from build123d import *

# Parameters (mm, degrees)
SKETCH_1_R             = 5.25
SM_BASE_FLANGE_1_DEPTH = 6


# Sheet-metal steps are written as plain solids
with BuildPart() as part:
    # Sketch 1 → Базовая кромка1 (new body)
    with BuildSketch(Plane.XY):
        Polygon((-41, -132.5), (-56, -117.5), (-56, 5), (-41, 20), (41, 20), (56, 5), (56, -117.5), (41, -132.5), align=None)
        with Locations((28, -61.72618932)):
            Circle(SKETCH_1_R, mode=Mode.SUBTRACT)
        with Locations((28, -92.5)):
            Circle(SKETCH_1_R, mode=Mode.SUBTRACT)
        with Locations((-28, -92.5)):
            Circle(SKETCH_1_R, mode=Mode.SUBTRACT)
        with Locations((-28, -61.72618932)):
            Circle(SKETCH_1_R, mode=Mode.SUBTRACT)
    extrude(amount=-SM_BASE_FLANGE_1_DEPTH)


solid = part.part
Source: CAD feature listing. Evaluate the final solid. Frame: model axes, mm. Coordinates: 2 decimals unless noted, no trailing zeros. Loops run counter-clockwise (first coordinate to the right, second up) from the corner with the lowest first, then second, coordinate; pieces in that order, holes last. Notation, with made-up numbers: (3, 6) - (24, 6) arc R14 cw to (24, 14) - close; hole circle Ø8 at (86, 10). An arc over 180 degrees is marked (long way). One line per item, written item: value. Start each with the question number.
1. Section B-B (y = -92.5). Return the cut outline in (x, z).
2. Section A-A (x = -28). Return the cut outline in (y, z).
3. Mould query, pull axis Y, two halves, no side actions, for faces 1 (the flat face through (-49, 12, -3)), 2 (the flat face through (48.6, -124.9, -3)), 3 (the flat face through (1, -55, 0)), 4 (the cylindrical face through (27.32, -56.52, -2.96)). Classes: pulls with the +Y half, pulls with the -Y half, needs draft (parallel to the pull), parting line crosses it, or undercut.
4. Section C-C (z = -2.9). Return the cut outline in (x, y), and give its area (3 significant figures).
5. Ray query, L1, parallel to Y at x = 28, z = -1.7; L2, parallel to Y at x = -29.5, z = -2.7; L3, parallel to X at y = -60, z = -0.3. Return the intervals inside material, ascending.
6. Section D-D (x = 45.5). Return the cut outline in (y, z), and give its area (3 significant figures).
Verdict:
1. outline: (-56, -6) - (-33.25, -6) - (-33.25, 0) - (-56, 0) - close; (-22.75, -6) - (22.75, -6) - (22.75, 0) - (-22.75, 0) - close; (33.25, -6) - (56, -6) - (56, 0) - (33.25, 0) - close
2. outline: (-132.5, -6) - (-97.75, -6) - (-97.75, 0) - (-132.5, 0) - close; (-87.25, -6) - (-66.98, -6) - (-66.98, 0) - (-87.25, 0) - close; (-56.48, -6) - (20, -6) - (20, 0) - (-56.48, 0) - close
3. face 1: pulls with the +Y half
3. face 2: pulls with the -Y half
3. face 3: needs draft
3. face 4: undercut
4. outline: (-56, -117.5) - (-41, -132.5) - (41, -132.5) - (56, -117.5) - (56, 5) - (41, 20) - (-41, 20) - (-56, 5) - close; hole circle Ø10.5 at (-28, -92.5); hole circle Ø10.5 at (-28, -61.73); hole circle Ø10.5 at (28, -92.5); hole circle Ø10.5 at (28, -61.73)
4. area: 16,300 mm2
5. L1: y = -132.5 to -97.75, -87.25 to -66.98, -56.48 to 20
5. L2: y = -132.5 to -97.53, -87.47 to -66.76, -56.7 to 20
5. L3: x = -56 to -32.96, -23.04 to 23.04, 32.96 to 56
6. outline: (-128, -6) - (15.5, -6) - (15.5, 0) - (-128, 0) - close
6. area: 861 mm2
